Can you work these out from the model? Positions are in its coordinate system, mm. A direction names the side the tool comes from. Round coordinates to 2 decimals unless told otherwise and drop trailing zeros. Loops run counter-clockwise (first coordinate to the right, second up) from the corner with the lowest first, then second, coordinate; pieces in that order, holes last. Notation, with made-up numbers: (49, 18.25) -> (85, 18.25) arc R17 cw to (85, 46.25) -> close; hole circle Ø2 at (-25.75, 38.25). An arc over 180 degrees is marked (long way). Use a Markdown table: item, result.
from build123d import *

# Parameters (mm, degrees)
SKETCH_1_W          = 380
SKETCH_1_H          = 115
EXTRUDE_1_DEPTH     = 20
SKETCH_2_R          = 8.5
CUT_EXTRUDE_1_DEPTH = 20
CHAMFER_1_SIZE      = 3
SKETCH_3_W          = 50
SKETCH_3_H          = 60
CUT_EXTRUDE_2_DEPTH = 200.515037027
CHAMFER_2_SIZE      = 8


with BuildPart() as part:
    # 草图1 → 凸台-拉伸1 (new body)
    with BuildSketch(Plane.XY):
        Rectangle(SKETCH_1_W, SKETCH_1_H)
    extrude(amount=EXTRUDE_1_DEPTH)

    # 草图2 → 切除-拉伸1 (cut)
    with BuildSketch(Plane.XY.offset(20)):
        with Locations((172, 0)):
            Circle(SKETCH_2_R)
    extrude(amount=-CUT_EXTRUDE_1_DEPTH, mode=Mode.SUBTRACT)

    # 倒角1
    chamfer_1_edges = [part.edges().sort_by_distance(p)[0] for p in [
        (190, 0, 20),
        (190, 0, 0),
    ]]
    chamfer(chamfer_1_edges, length=CHAMFER_1_SIZE)

    # 草图3 → 切除-拉伸2 (cut, through all)
    with BuildSketch(Plane.XY.offset(20)):
        with Locations((-165, 0)):
            Rectangle(SKETCH_3_W, SKETCH_3_H)
    extrude(amount=-CUT_EXTRUDE_2_DEPTH, mode=Mode.SUBTRACT)

    # 倒角2
    chamfer_2_edges = [part.edges().sort_by_distance(p)[0] for p in [
        (-1.5, 57.5, 20),
        (-1.5, 57.5, 0),
        (-1.5, -57.5, 0),
        (-1.5, -57.5, 20),
    ]]
    chamfer(chamfer_2_edges, length=CHAMFER_2_SIZE)


solid = part.part
1. I want a section at B-B (x = 172). Please give me the cut outline in (y, z).
Answer sheet:
| item | result |
|---|---|
| outline | (-57.5, 8) -> (-49.5, 0) -> (-8.5, 0) -> (-8.5, 20) -> (-49.5, 20) -> (-57.5, 12) -> close; (8.5, 0) -> (49.5, 0) -> (57.5, 8) -> (57.5, 12) -> (49.5, 20) -> (8.5, 20) -> close |
2. I need wall thicknesses on line 1 (Y direction, x = -149.5, z = 17); line 2 (X direction, y = 27, z = 7); line 3 (Y direction, x = 172, z = 15). Which ranges of each line are inside material? Lowest first, please.
Answer sheet:
| item | result |
|---|---|
| line 1 | y = -52.5 to -30, 30 to 52.5 |
| line 2 | x = -140 to 190 |
| line 3 | y = -54.5 to -8.5, 8.5 to 54.5 |
3. I want a section at A-A (y = 4). Please give me the cut outline in (x, z), plus the area to 3 significant figures.
Answer sheet:
| item | result |
|---|---|
| outline | (-140, 0) -> (164.5, 0) -> (164.5, 20) -> (-140, 20) -> close; (179.5, 0) -> (187, 0) -> (190, 3) -> (190, 17) -> (187, 20) -> (179.5, 20) -> close |
| area | 6,290 mm² |
4. Which directions (+Z, -Z, +X, -X, +Y, -Y) give clear straight access to the entire face, cutting with the end or side of a thin tool? Please do faces 1 (the flat face through (-2.7, 53.6, 4.1)), 2 (the flat face through (-140, 0, 10)).
Answer sheet:
| item | result |
|---|---|
| face 1 | -Z, +X, -X, +Y |
| face 2 | +Z, -Z, -X |
5. I want a section at D-D (x = 44.5). Please give me the cut outline in (y, z), plus the area to 3 significant figures.
Answer sheet:
| item | result |
|---|---|
| outline | (-57.5, 8) -> (-49.5, 0) -> (49.5, 0) -> (57.5, 8) -> (57.5, 12) -> (49.5, 20) -> (-49.5, 20) -> (-57.5, 12) -> close |
| area | 2,170 mm² |
6. Will these pins go through, and if not, where does the flat tip stop? pin 1 Ø4 at (x, z) = (21.5, 2.5) entering from +Y; pin 2 Ø2 at (x, z) = (-109.5, 15.5) entering from +Y; pin 3 Ø15.5 at (x, y) = (172, 0) entering from +Z; pin 4 Ø8 at (y, z) = (11.5, 4) entering from -X.
Answer sheet:
| item | result |
|---|---|
| pin 1 | stops at y = 54 |
| pin 2 | stops at y = 55 |
| pin 3 | passes through |
| pin 4 | stops at x = -140 |
7. I want a section at C-C (y = 26). Please give me the cut outline in (x, z), plus the area to 3 significant figures.
Answer sheet:
| item | result |
|---|---|
| outline | (-140, 0) -> (187, 0) -> (190, 3) -> (190, 17) -> (187, 20) -> (-140, 20) -> close |
| area | 6,590 mm² |
8. If we mould it in two halves opening along Y, with no side actions, what happens to faces 3 (the flat face through (-165, 30, 10)), 4 (the flat face through (-4, 1, 0)), 5 (the flat face through (-165, -30, 10)), 6 (the flat face through (-2.7, 53.6, 15.9))? For each: +Y half, -Y half, draft (parallel to the pull), parting line (faces both ways), or undercut.
Answer sheet:
| item | result |
|---|---|
| face 3 | undercut |
| face 4 | draft |
| face 5 | undercut |
| face 6 | +Y half |
